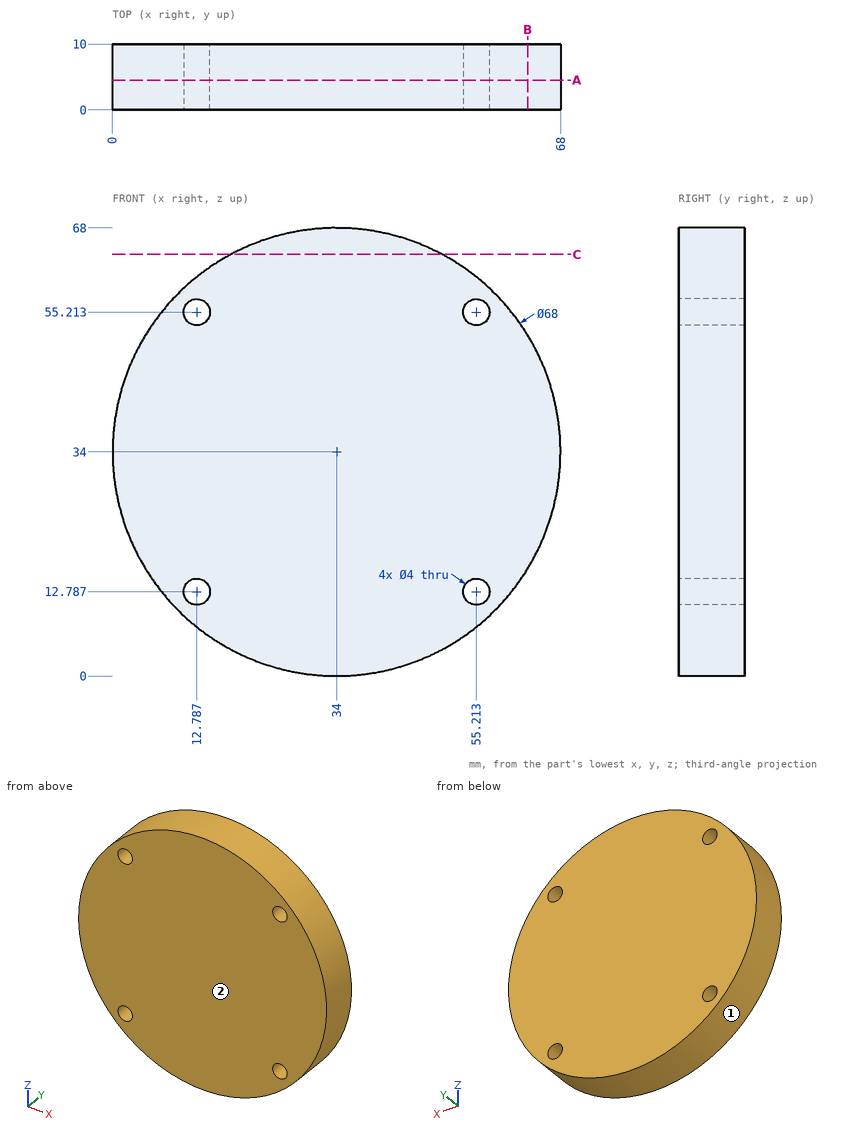
Study the drawing (mm; zero at the part's minimum x, y, z) and answer. Give positions to 0.01 mm unless a question says otherwise; leave off trailing zeros. Loops run counter-clockwise (first coordinate to the right, second up) from the corner with the lowest first, then second, coordinate; pieces in that order, holes last. Notation, with made-up numbers: (17.5, -4.75) - (76.5, -4.75) arc R36 ccw to (76.5, 34.25) - close; hole circle Ø8 at (60.5, -38.5). An arc over 180 degrees is marked (long way). Return JSON: item names as keys, results as strings. Group by question number.
1. Given pin 1 Ø3.5 at (x, z) = (55.21, 12.79) entering from -Y (3 decimals); pin 2 Ø2 at (y, z) = (6, 52) entering from -X (1 decimal); pin 3 Ø5 at (y, z) = (8.5, 11.5) entering from +X (1 decimal), each flat-ended and moving along its own axis, determine where each tip first touches the part or whether it passes through.
2. Find section B-B (x = 63). Write down the section's boundary in (y, z), then the cut area to 3 significant figures.
3. Determine the mould class of the marked faces 1 and 2 for opening direction Z: pulls with the +Z half, pulls with the -Z half, needs draft (parallel to the pull), parting line crosses it, or undercut.
4. Find section A-A (y = 4.5). Write down the section's boundary in (x, z), then the cut area to 3 significant figures.
5. Find section C-C (z = 64). Write down the section's boundary in (x, y).
6. Straight lines are drawn through the part: line 1 (Z direction, x = 13.5, y = 8.75) (1 decimal); line 2 (Z direction, x = 23, y = 7.25). For each, find the intervals that lie inside material, in ascending order. Write a range as [from, to].
Verdict:
{
 "1": {"pin 1": "passes through", "pin 2": "stops at x = 4.6", "pin 3": "stops at x = 61.5"},
 "2": {"outline": "(0, 16.25) - (10, 16.25) - (10, 51.75) - (0, 51.75) - close", "area": "355 mm^2"},
 "3": {"face 1": "parting line crosses it", "face 2": "needs draft"},
 "4": {"outline": "circle Ø68 at (34, 34); hole circle Ø4 at (12.79, 12.79); hole circle Ø4 at (12.79, 55.21); hole circle Ø4 at (55.21, 12.79); hole circle Ø4 at (55.21, 55.21)", "area": "3,580 mm^2"},
 "5": {"outline": "(18, 0) - (50, 0) - (50, 10) - (18, 10) - close"},
 "6": {"line 1": "z = [6.9, 10.9], [14.7, 53.3], [57.1, 61.1]", "line 2": "z = [1.83, 66.17]"}
}
